from build123d import *

# Parameters (mm, degrees)
BODY_DEPTH          = 30
SKETCH2_R           = 7.5
ROTATING_PIN_DEPTH  = 50
SKETCH3_R           = 7.5
BOSS_EXTRUDE3_DEPTH = 50
SKETCH4_W           = 10
SKETCH4_H           = 100
BOSS_EXTRUDE4_DEPTH = 230
SKETCH5_R           = 7.5
BOSS_EXTRUDE5_DEPTH = 50
SKETCH6_R           = 3.378341257
CUT_EXTRUDE1_DEPTH  = 10


with BuildPart() as part:
    # Sketch1 → body (new body)
    with BuildSketch(Plane(origin=(0, 0, 0), x_dir=(1, 0, 0), z_dir=(0, 1, 0))):
        Polygon((0, 0), (200, 0), (200, 230), (190, 230), (190, 10), (0, 10), align=None)
    extrude(amount=BODY_DEPTH)

    # Sketch2 → rotating pin (add)
    with BuildSketch(Plane(origin=(0, 0, -10), x_dir=(-1, 0, 0), z_dir=(0, 0, -1))):
        with Locations((-7.5, 15)):
            Circle(SKETCH2_R)
    extrude(amount=ROTATING_PIN_DEPTH)

    # Sketch3 → Boss-Extrude3 (add)
    with BuildSketch(Plane.ZY.offset(-190)):
        with Locations(Location((-222.5, 15, 0), (0, 0, 180))):
            Circle(SKETCH3_R)
    extrude(amount=BOSS_EXTRUDE3_DEPTH)

    # Sketch4 → Boss-Extrude4 (add, through all)
    with BuildSketch(Plane.XY):
        with Locations((195, -20)):
            Rectangle(SKETCH4_W, SKETCH4_H)
    extrude(amount=-BOSS_EXTRUDE4_DEPTH)

    # Sketch5 → Boss-Extrude5 (add)
    with BuildSketch(Plane.ZY.offset(-190)):
        with Locations(Location((-222.5, -55, 0), (0, 0, 180))):
            Circle(SKETCH5_R)
    extrude(amount=BOSS_EXTRUDE5_DEPTH)

    # Sketch6 → Cut-Extrude1 (cut)
    with BuildSketch(Plane(origin=(0, 30, 0), x_dir=(1, 0, 0), z_dir=(0, 1, 0))):
        with Locations(Location((7.831461534, 4.216291967, 0), (0, 0, 270))):
            Circle(SKETCH6_R)
    extrude(amount=-CUT_EXTRUDE1_DEPTH, mode=Mode.SUBTRACT)


solid = part.part
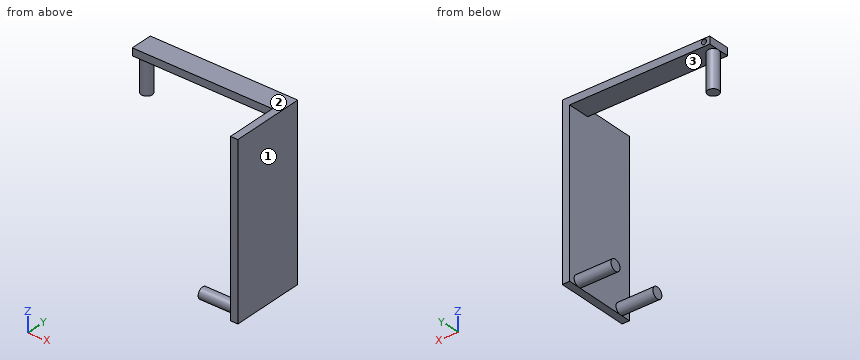
For this review, take the finished solid that the model builds, in its own axes (mm). Face numbers are marked on the shaded views. Round coordinates to 2 decimals unless told otherwise and drop trailing zeros. Loops run counter-clockwise (first coordinate to the right, second up) from the corner with the lowest first, then second, coordinate; pieces in that order, holes last. Notation, with made-up numbers: (76, 56.5) - (103, 56.5) arc R10 cw to (103, 75.5) - close; hole circle Ø2 at (-24.75, -30). An arc over 180 degrees is marked (long way). One line per item, written item: value. Start each with the question number.
Item 1: Clearance check with flat-ended pins moving along their axes: pin 1 Ø7.5 at (y, z) = (18.5, -221) entering from -X; pin 2 Ø1 at (y, z) = (-42, -197.5) entering from -X; pin 3 Ø8 at (x, y) = (112, 19.5) entering from -Z. State where each tip first meets the part, or that it passes through.
Item 2: For L1, parallel to X at y = 8.5, z = -97; L2, parallel to Z at x = 55.5, y = 16.5; L3, parallel to Z at x = 173, y = 13, list the stretches that pass through material, from the lowest coordinate up.
Item 3: Take a section at A-A (x = 166). Give the boundary of the cut face in (y, z), plus the area to 3 significant figures.
Item 4: Take a section at B-B (z = -47.5). Give the boundary of the cut face in (x, y), plus the area to 3 significant figures.
Item 5: Take a section at D-D (y = -29). Give the boundary of the cut face in (x, z), plus the area to 3 significant figures.
Item 6: The part is to be moulded in two halves that separate along X. For the marked faces 1, 2 and 3, say which applies: +X half, -X half, draft (parallel to the pull), parting line (faces both ways), or undercut.
Item 7: Take a section at C-C (z = -96.5). Give the boundary of the cut face in (x, y), plus the area to 3 significant figures.
Answer below:
1. pin 1: stops at x = 140
1. pin 2: stops at x = 190
1. pin 3: stops at z = -10
2. L1: x = 190 to 200
2. L2: z = -10 to 0
2. L3: z = -229.73 to -215.27, -10 to 0
3. outline: circle Ø15 at (-55, -222.5); (0, -10) - (30, -10) - (30, 0) - (0, 0) - close; circle Ø15 at (15, -222.5)
3. area: 653 mm2
4. outline: circle Ø15 at (7.5, 15); (190, -70) - (200, -70) - (200, 30) - (190, 30) - close
4. area: 1,180 mm2
5. outline: (190, -230) - (200, -230) - (200, 0) - (190, 0) - close
5. area: 2,300 mm2
6. face 1: +X half
6. face 2: draft
6. face 3: undercut
7. outline: (190, -70) - (200, -70) - (200, 30) - (190, 30) - close
7. area: 1,000 mm2
